For this review, take the finished solid that the model builds, in its own axes (mm). A direction names the side the tool comes from. Round coordinates to 2 decimals unless told otherwise and drop trailing zeros. Order: outer loops, then holes, each group sorted by start corner. A loop starts at its lowest first (then second) coordinate and runs counter-clockwise, first axis right, second up. Notation, with made-up numbers: (15.25, 11) -> (34.25, 11) arc R15 cw to (34.25, 29) -> close; hole circle Ø9 at (34, 79.25). An arc over 180 degrees is marked (long way). Use a Markdown table: item, result. Add a question column.
1) Clearance check with flat-ended pins moving along their axes: P1, Ø1.5, axis at x = 0.5, z = 15, coming from the -Y side; P2, Ø6, axis at x = 7, z = 57.5, coming from the +Y side (3 decimals); P3, Ø1.9, axis at y = 16, z = 24.5, coming from the +X side. State where each tip first meets the part, or that it passes through.
2) Draft analysis for pull direction Y (two halves, no side actions). For faces 1 (the face through (14, -7, 88)), 2 (the face through (-5, 16, 43)), 3 (the face through (0.59, -14.99, 43.38)), 4 (the face through (-4.101, 31.232, 43.384)), state which applies: pulls with the +Y half, pulls with the -Y half, needs draft (parallel to the pull), parting line crosses it, or undercut.
3) Consider section D-D (x = 22). State the section outline as (y, z) points, plus the area to 3 significant figures.
4) Wall thickness on line 1 along Y through (x, z) = (0, 67); line 2 along Y through (x, z) = (1.5, 79); line 3 along X through (y, z) = (-11.5, 72.5): over which ranges is each line inside the solid? List them lowest first. Write a range as [from, to].
5) Consider section C-C (z = 68.5). State the section outline as (x, y) points, plus the area to 3 significant figures.
6) Consider section A-A (x = 0). State the section outline as (y, z) points, plus the area to 3 significant figures.
7) Machinability: for faces 5 (the face through (5, 16, 43)), 6 (the face through (14, -7, 0)), which of the approach directions +Z, -Z, +X, -X, +Y, -Y give a long, thin tool a straight path to every point of the face, cutting with its end or side? Answer none if there is none.
8) Consider section B-B (y = 0). State the section outline as (x, z) points.
```python
from build123d import *

# Parameters (mm, degrees)
SKETCH1_R           = 31.5
BOSS_EXTRUDE1_DEPTH = 88


with BuildPart() as part:
    # Sketch1 → Boss-Extrude1 (new body)
    with BuildSketch(Plane.XY):
        Circle(SKETCH1_R)
        with BuildLine():
            Line((-5, 18), (5, 18))
            Line((5, 18), (5, 14.142135624))
            ThreePointArc((5, 14.142135624), (0, -15), (-5, 14.142135624))
            Line((-5, 14.142135624), (-5, 18))
        make_face(mode=Mode.SUBTRACT)
    extrude(amount=BOSS_EXTRUDE1_DEPTH)


solid = part.part
```
Results list:
| question | item | result |
|---|---|---|
| 1 | P1 | y = -31.5 |
| 1 | P2 | y = 31.245 |
| 1 | P3 | x = 27.67 |
| 2 | face 1 | needs draft |
| 2 | face 2 | undercut |
| 2 | face 3 | undercut |
| 2 | face 4 | parting line crosses it |
| 3 | outline | (-22.54, 0) -> (22.54, 0) -> (22.54, 88) -> (-22.54, 88) -> close |
| 3 | area | 3,970 mm2 |
| 4 | line 1 | [-31.5, -15], [18, 31.5] |
| 4 | line 2 | [-31.46, -14.92], [18, 31.46] |
| 4 | line 3 | [-29.33, -9.63], [9.63, 29.33] |
| 5 | outline | circle Ø63 at (0, 0); hole (-5, 14.14) arc R15 ccw (long way) to (5, 14.14) -> (5, 18) -> (-5, 18) -> close |
| 5 | area | 2,380 mm2 |
| 6 | outline | (-31.5, 0) -> (-15, 0) -> (-15, 88) -> (-31.5, 88) -> close; (18, 0) -> (31.5, 0) -> (31.5, 88) -> (18, 88) -> close |
| 6 | area | 2,640 mm2 |
| 7 | face 5 | +Z, -Z |
| 7 | face 6 | -Z, +X, -X, +Y, -Y |
| 8 | outline | (-31.5, 0) -> (-15, 0) -> (-15, 88) -> (-31.5, 88) -> close; (15, 0) -> (31.5, 0) -> (31.5, 88) -> (15, 88) -> close |
